from build123d import *

# Parameters (mm, degrees)
SKETCH1_W           = 150
SKETCH1_H           = 140
BOSS_EXTRUDE1_DEPTH = 86
SKETCH2_R           = 1.5
CUT_EXTRUDE1_DEPTH  = 3
BOTTOM_VENT_W       = 128.112390575
BOTTOM_VENT_H       = 30.300850467
CUT_EXTRUDE2_DEPTH  = 3
SKETCH4_R           = 14
BOSS_EXTRUDE2_DEPTH = 52
SKETCH5_W           = 98.859747303
SKETCH5_H           = 72.009781986
CUT_EXTRUDE3_DEPTH  = 3


with BuildPart() as part:
    # Sketch1 → Boss-Extrude1 (new body)
    with BuildSketch(Plane(origin=(0, 0, 0), x_dir=(1, 0, 0), z_dir=(0, 1, 0))):
        with Locations((75, 70)):
            Rectangle(SKETCH1_W, SKETCH1_H)
    extrude(amount=BOSS_EXTRUDE1_DEPTH)

    # Sketch2 → Cut-Extrude1 (cut)
    with BuildSketch(Plane.XY):
        with Locations((6, 80)):
            Circle(SKETCH2_R)
        with Locations((6, 16)):
            Circle(SKETCH2_R)
        with Locations((120, 6)):
            Circle(SKETCH2_R)
        with Locations((144, 80)):
            Circle(SKETCH2_R)
    extrude(amount=-CUT_EXTRUDE1_DEPTH, mode=Mode.SUBTRACT)

    # bottom vent → Cut-Extrude2 (cut)
    with BuildSketch(Plane(origin=(0, 86, 0), x_dir=(1, 0, 0), z_dir=(0, 1, 0))):
        with Locations((76.529847499, 114.217527718)):
            Rectangle(BOTTOM_VENT_W, BOTTOM_VENT_H)
    extrude(amount=-CUT_EXTRUDE2_DEPTH, mode=Mode.SUBTRACT)

    # Sketch4 → Boss-Extrude2 (add)
    with BuildSketch(Plane(origin=(0, 0, -140), x_dir=(-1, 0, 0), z_dir=(0, 0, -1))):
        with Locations((-133.5, 66)):
            Circle(SKETCH4_R)
    extrude(amount=BOSS_EXTRUDE2_DEPTH)

    # Sketch5 → Cut-Extrude3 (cut)
    with BuildSketch(Plane(origin=(0, 0, -140), x_dir=(-1, 0, 0), z_dir=(0, 0, -1))):
        with Locations((-65.179614688, 41.905186472)):
            Rectangle(SKETCH5_W, SKETCH5_H)
    extrude(amount=-CUT_EXTRUDE3_DEPTH, mode=Mode.SUBTRACT)


solid = part.part
Design review of the part built by this model. Coordinates are the model's own, in mm. A direction names the side the tool comes from. Round coordinates to 2 decimals unless told otherwise and drop trailing zeros. Write each loop counter-clockwise with the first axis right and the second up, starting at its lowest first coordinate (ties: lowest second). Pieces come first, ordered by that corner, then holes.
Item 1: Wall thickness on L1, parallel to Y at x = 6, z = -1; L2, parallel to X at y = 80, z = -1.1; L3, parallel to Z at x = 33.5, y = 80.5: over which ranges is each line inside the solid? List them lowest first.
Item 2: Draft analysis for pull direction X (two halves, no side actions). For faces 1 (the flat face through (76, 83, -114)), 2 (the cylindrical face through (135.32, 79.88, -165.64)), 3 (the flat face through (74, 4, -140)), state which applies: released by +X, released by -X, zero draft, split by the parting line, or undercut.
Item 3: Consider section C-C on x = 133.5. Give the boundary of the cut face in (y, z).
Item 4: For faces 4 (the flat face through (66, 42, -137)), 5 (the flat face through (74, 86, -55)), list the 3-axis set-ups (+Z, -Z, +X, -X, +Y, -Y) from which the entire face can be reached by the end or side of a thin tool; tool diameter is ignored.
Item 5: Consider section B-B on y = 66. Give the boundary of the cut face in (x, z), and give its area (3 significant figures).
Item 6: Consider section A-A on z = -117.5. Give the boundary of the cut face in (x, y), and give its area (3 significant figures).
Item 7: For pin 1 Ø3.5 at (x, y) = (144, 80) entering from +Z; pin 2 Ø2.5 at (x, y) = (6, 80) entering from +Z; pin 3 Ø8 at (x, y) = (52.5, 24) entering from -Z; pin 4 Ø1.8 at (x, y) = (6, 16) entering from -Z, all flat-tipped, find the tip position at first contact; note any pin that passes through.
Check values:
1. L1: y = 0 to 14.5, 17.5 to 78.5, 81.5 to 86
1. L2: x = 0 to 4.5, 7.5 to 142.5, 145.5 to 150
1. L3: z = -140 to 0
2. face 1: undercut
2. face 2: split by the parting line
2. face 3: zero draft
3. outline: (0, -140) - (52, -140) - (52, -192) - (80, -192) - (80, -140) - (86, -140) - (86, -129.37) - (83, -129.37) - (83, -99.07) - (86, -99.07) - (86, 0) - (0, 0) - close
4. face 4: -Z
4. face 5: +Z, -Z, +X, -X, +Y
5. outline: (0, -140) - (15.75, -140) - (15.75, -137) - (114.61, -137) - (114.61, -140) - (119.5, -140) - (119.5, -192) - (147.5, -192) - (147.5, -140) - (150, -140) - (150, 0) - (0, 0) - close
5. area: 22,200 mm2
6. outline: (0, 0) - (150, 0) - (150, 86) - (140.59, 86) - (140.59, 83) - (12.47, 83) - (12.47, 86) - (0, 86) - close
6. area: 12,500 mm2
7. pin 1: stops at z = 0
7. pin 2: stops at z = -3
7. pin 3: stops at z = -137
7. pin 4: stops at z = -140
